Input: part model. Units: mm. Frame: model coordinates. Coordinates: 2 decimals unless noted, no trailing zeros. Loops run counter-clockwise (first coordinate to the right, second up) from the corner with the lowest first, then second, coordinate; pieces in that order, holes last. Notation, with made-up numbers: (-13, -19) - (9, -19) arc R8 ccw to (9, -7) - close; hole circle Ø4 at (-37, 28.5). An arc over 180 degrees is marked (long way). Use one line per item in the form item = value.
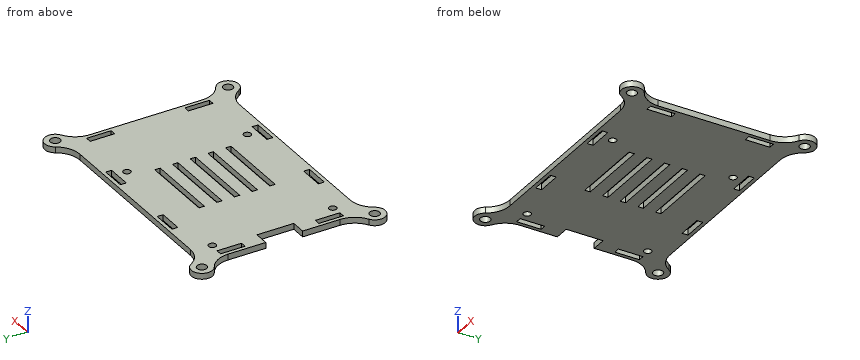
from build123d import *

# Parameters (mm, degrees)
F0_R     = 2
F0_W     = 2.4
F0_H     = 10
F0_R_2   = 1.5
F0_W_2   = 10
F0_H_2   = 2.4
F0_W_3   = 30
F0_H_3   = 2.2
F1_DEPTH = 2.4


with BuildPart() as f1:
    # F0 (on Top) → F1 (new body)
    with BuildSketch(Plane.XY):
        with BuildLine():
            ThreePointArc((46.111466, 37.36014), (42.463054, 33.799465), (37.533481, 32.5))
            Line((37.533481, 32.5), (-37.533481, 32.5))
            ThreePointArc((-37.533481, 32.5), (-42.463054, 33.799465), (-46.111466, 37.36014))
            ThreePointArc((-46.111466, 37.36014), (-52.859026, 38.171979), (-51.965035, 31.434812))
            ThreePointArc((-51.965035, 31.434812), (-48.329658, 27.777326), (-47, 22.794839))
            Line((-47, 22.794839), (-47, 7.5))
            Line((-47, 7.5), (-41, 7.5))
            Line((-41, 7.5), (-41, -7.5))
            Line((-41, -7.5), (-47, -7.5))
            Line((-47, -7.5), (-47, -22.794839))
            ThreePointArc((-47, -22.794839), (-48.329658, -27.777326), (-51.965035, -31.434812))
            ThreePointArc((-51.965035, -31.434812), (-52.859026, -38.171979), (-46.111466, -37.36014))
            ThreePointArc((-46.111466, -37.36014), (-42.463054, -33.799465), (-37.533481, -32.5))
            Line((-37.533481, -32.5), (37.533481, -32.5))
            ThreePointArc((37.533481, -32.5), (42.463054, -33.799465), (46.111466, -37.36014))
            ThreePointArc((46.111466, -37.36014), (52.859026, -38.171979), (51.965035, -31.434812))
            ThreePointArc((51.965035, -31.434812), (48.329658, -27.777326), (47, -22.794839))
            Line((47, -22.794839), (47, 22.794839))
            ThreePointArc((47, 22.794839), (48.329658, 27.777326), (51.965035, 31.434812))
            ThreePointArc((51.965035, 31.434812), (52.859026, 38.171979), (46.111466, 37.36014))
        make_face()
        with Locations((-49.8, -35.15)):
            Circle(F0_R, mode=Mode.SUBTRACT)
        with Locations((-44.3, -20)):
            Rectangle(F0_W, F0_H, mode=Mode.SUBTRACT)
        with Locations((-39.1, -24.5)):
            Circle(F0_R_2, mode=Mode.SUBTRACT)
        with Locations((-17.5, -29.8)):
            Rectangle(F0_W_2, F0_H_2, mode=Mode.SUBTRACT)
        with Locations((17.5, -29.8)):
            Rectangle(F0_W_2, F0_H_2, mode=Mode.SUBTRACT)
        with Locations((18.9, -24.5)):
            Circle(F0_R_2, mode=Mode.SUBTRACT)
        with Locations((49.8, -35.15)):
            Circle(F0_R, mode=Mode.SUBTRACT)
        with Locations((44.3, -20)):
            Rectangle(F0_W, F0_H, mode=Mode.SUBTRACT)
        with Locations((0, -14.4)):
            Rectangle(F0_W_3, F0_H_3, mode=Mode.SUBTRACT)
        with Locations((0, -7.2)):
            Rectangle(F0_W_3, F0_H_3, mode=Mode.SUBTRACT)
        with Locations((-44.3, 20)):
            Rectangle(F0_W, F0_H, mode=Mode.SUBTRACT)
        with Locations((-39.1, 24.5)):
            Circle(F0_R_2, mode=Mode.SUBTRACT)
        with Locations((-49.8, 35.15)):
            Circle(F0_R, mode=Mode.SUBTRACT)
        with Locations((-17.5, 29.8)):
            Rectangle(F0_W_2, F0_H_2, mode=Mode.SUBTRACT)
        Rectangle(F0_W_3, F0_H_3, mode=Mode.SUBTRACT)
        with Locations((0, 7.2)):
            Rectangle(F0_W_3, F0_H_3, mode=Mode.SUBTRACT)
        with Locations((0, 14.4)):
            Rectangle(F0_W_3, F0_H_3, mode=Mode.SUBTRACT)
        with Locations((18.9, 24.5)):
            Circle(F0_R_2, mode=Mode.SUBTRACT)
        with Locations((17.5, 29.8)):
            Rectangle(F0_W_2, F0_H_2, mode=Mode.SUBTRACT)
        with Locations((44.3, 20)):
            Rectangle(F0_W, F0_H, mode=Mode.SUBTRACT)
        with Locations((49.8, 35.15)):
            Circle(F0_R, mode=Mode.SUBTRACT)
    extrude(amount=F1_DEPTH)


solid = f1.part
Q1. Cut plane C-C, the plane x = 18.9. Return loops of the section in (y, z), then the cut area to 3 significant figures.
Check values:
outline = (-32.5, 0) - (-31, 0) - (-31, 2.4) - (-32.5, 2.4) - close; (-28.6, 0) - (-26, 0) - (-26, 2.4) - (-28.6, 2.4) - close; (-23, 0) - (23, 0) - (23, 2.4) - (-23, 2.4) - close; (26, 0) - (28.6, 0) - (28.6, 2.4) - (26, 2.4) - close; (31, 0) - (32.5, 0) - (32.5, 2.4) - (31, 2.4) - close
area = 130 mm²
Q2. Cut plane D-D, the plane y = 35.15. Return loops of the section in (x, z).
Check values:
outline = (-54.1, 0) - (-51.8, 0) - (-51.8, 2.4) - (-54.1, 2.4) - close; (-47.8, 0) - (-44.31, 0) - (-44.31, 2.4) - (-47.8, 2.4) - close; (44.31, 0) - (47.8, 0) - (47.8, 2.4) - (44.31, 2.4) - close; (51.8, 0) - (54.1, 0) - (54.1, 2.4) - (51.8, 2.4) - close
Q3. Cut plane B-B, the plane y = 18.5. Return loops of the section in (x, z).
Check values:
outline = (-47, 0) - (-45.5, 0) - (-45.5, 2.4) - (-47, 2.4) - close; (-43.1, 0) - (43.1, 0) - (43.1, 2.4) - (-43.1, 2.4) - close; (45.5, 0) - (47, 0) - (47, 2.4) - (45.5, 2.4) - close
Q4. Cut plane A-A, the plane x = -5. Return loops of the section in (y, z).
Check values:
outline = (-32.5, 0) - (-15.5, 0) - (-15.5, 2.4) - (-32.5, 2.4) - close; (-13.3, 0) - (-8.3, 0) - (-8.3, 2.4) - (-13.3, 2.4) - close; (-6.1, 0) - (-1.1, 0) - (-1.1, 2.4) - (-6.1, 2.4) - close; (1.1, 0) - (6.1, 0) - (6.1, 2.4) - (1.1, 2.4) - close; (8.3, 0) - (13.3, 0) - (13.3, 2.4) - (8.3, 2.4) - close; (15.5, 0) - (32.5, 0) - (32.5, 2.4) - (15.5, 2.4) - close
Q5. First-contact query: P1, Ø1.1, axis at y = 7, z = 1, coming from the -X side; P2, Ø0.7, axis at y = 7.5, z = 0.5, coming from the +X side; P3, Ø1.2, axis at x = -20, z = 1, coming from the +Y side. Flat tips, straight axial feed; report the tip coordinate or a pass-through.
Check values:
P1 = -47
P2 = 47
P3 = 32.5
Q6. Ray query, line 1 along Y through (x, z) = (15.5, 2.3); line 2 along Y through (x, z) = (-1, 1.9); line 3 along X through (y, z) = (6.5, 1.8). Return the intervals inside material, ascending. Write a range as [from, to].
Check values:
line_1 = [-32.5, -31], [-28.6, 28.6], [31, 32.5]
line_2 = [-32.5, -15.5], [-13.3, -8.3], [-6.1, -1.1], [1.1, 6.1], [8.3, 13.3], [15.5, 32.5]
line_3 = [-41, -15], [15, 47]
